Work out the finished part from the listing and answer in its coordinate system (mm). A direction names the side the tool comes from. Round coordinates to 2 decimals unless told otherwise and drop trailing zeros. Write each loop counter-clockwise with the first axis right and the second up, starting at its lowest first coordinate (ties: lowest second). Pieces come first, ordered by that corner, then holes. Notation, with made-up numbers: (-32.5, 19) -> (21.5, 19) arc R19 ccw to (21.5, 35) -> close; hole circle Ø8 at (-27.5, 58.25). An arc over 180 degrees is marked (long way). Answer as a JSON object with one key per item and string values. Group by question number.
from build123d import *

# Parameters (mm, degrees)
F1_DEPTH = 19.05
F3_D     = 12.7
F5_D     = 12.7
F6_R     = 2.54


with BuildPart() as f1:
    # F0 (on Top) → F1 (new body)
    with BuildSketch(Plane.XY):
        Polygon((45.404016, -4.03813), (-1.694917, -4.03813), (-1.694917, 5.48687), (-33.444917, 5.48687), (-33.444917, -0.86313), (-7.148128, -0.86313), (-7.148128, -26.26313), (-33.444917, -26.26313), (-33.444917, -32.61313), (-1.694917, -32.61313), (-1.694917, -23.08813), (45.404016, -23.08813), align=None)
    extrude(amount=F1_DEPTH)

    # F3 (through all)
    with Locations(Plane.XZ.offset(32.61313)):
        with Locations((-23.919917, 9.525)):
            Hole(F3_D / 2)

    # F5 (through all)
    with Locations(Plane.XZ.offset(23.08813)):
        with Locations((35.879016, 9.525)):
            Hole(F5_D / 2)

    # F6
    f6_edges = [f1.edges().sort_by_distance(p)[0] for p in [
        (45.404016, -13.56313, 19.05),
        (45.404016, -13.56313, 0),
        (-7.148128, -13.56313, 19.05),
        (-7.148128, -13.56313, 0),
    ]]
    fillet(f6_edges, radius=F6_R)


solid = f1.part
1) A cutting plane is placed at C-C on y = -18. Determine the outline of the cut face in (x, z) (3 decimals), plus the area to 3 significant figures.
2) Each of these flat-tipped pins is pushed along its axis until it touches: P1, Ø5, axis at x = 25.5, z = 10, coming from the -Y side; P2, Ø7, axis at y = -9, z = 7, coming from the -X side; P3, Ø5.5, axis at x = -25, z = 8.5, coming from the +Y side; P4, Ø3, axis at y = -28, z = 13.5, coming from the +X side. Where does it stop, or does it pass through?
3) A cutting plane is placed at D-D on x = 20. Determine the outline of the cut face in (y, z).
4) A tool of negligible diameter and unlimited length cuts with its end or side. For faces 4 (the face through (-6.38, -13.74, 18.33)), 5 (the face through (22, -4.038, 9)), 6 (the face through (-1.695, -28, 9)), from which of +Z, -Z, +X, -X, +Y, -Y can it reach the whole face along a straight path? Write none if from no direction.
5) Straight lines are drawn through the part: L1, parallel to Y at x = -12, z = 1.5; L2, parallel to Y at x = 0.5, z = 16.5; L3, parallel to X at y = -21, z = 3.75. For each, find the intervals that lie inside material, in ascending order.
6) A cutting plane is placed at A-A on x = -15. Determine the outline of the cut face in (y, z), plus the area to 3 significant figures.
7) A cutting plane is placed at B-B on z = 13.5. Determine the outline of the cut face in (x, y).
8) For a pull along Y with two mould halves and no side action, classify faces 1 (the face through (-14, -32.613, 9)), 2 (the face through (-7.148, -13, 9)), 3 (the face through (44.68, -13.43, 0.764)) as released by +Y, released by -Y, zero draft, split by the parting line, or undercut.
Established:
{
 "1": {"outline": "(-7.148, 2.54) arc R2.54 ccw to (-4.608, 0) -> (42.864, 0) arc R2.54 ccw to (45.404, 2.54) -> (45.404, 16.51) arc R2.54 ccw to (42.864, 19.05) -> (-4.608, 19.05) arc R2.54 ccw to (-7.148, 16.51) -> close; hole circle Ø12.7 at (35.879, 9.525)", "area": "869 mm²"},
 "2": {"P1": "stops at y = -23.09", "P2": "stops at x = -7.15", "P3": "passes through", "P4": "stops at x = -1.69"},
 "3": {"outline": "(-23.09, 0) -> (-4.04, 0) -> (-4.04, 19.05) -> (-23.09, 19.05) -> close"},
 "4": {"face 4": "+Z, -X", "face 5": "+Z, -Z, +X, +Y", "face 6": "+Z, -Z, +X, -Y"},
 "5": {"L1": "y = -32.61 to -26.26, -0.86 to 5.49", "L2": "y = -23.09 to -4.04", "L3": "x = -7.15 to 33.24, 38.52 to 45.4"},
 "6": {"outline": "(-32.61, 0) -> (-26.26, 0) -> (-26.26, 19.05) -> (-32.61, 19.05) -> close; (-0.86, 0) -> (5.49, 0) -> (5.49, 19.05) -> (-0.86, 19.05) -> close", "area": "242 mm²"},
 "7": {"outline": "(-33.44, -32.61) -> (-28.87, -32.61) -> (-28.87, -26.26) -> (-33.44, -26.26) -> close; (-33.44, -0.86) -> (-28.87, -0.86) -> (-28.87, 5.49) -> (-33.44, 5.49) -> close; (-18.97, -32.61) -> (-1.69, -32.61) -> (-1.69, -23.09) -> (30.93, -23.09) -> (30.93, -4.04) -> (-1.69, -4.04) -> (-1.69, 5.49) -> (-18.97, 5.49) -> (-18.97, -0.86) -> (-7.15, -0.86) -> (-7.15, -26.26) -> (-18.97, -26.26) -> close; (40.83, -23.09) -> (45.4, -23.09) -> (45.4, -4.04) -> (40.83, -4.04) -> close"},
 "8": {"face 1": "released by -Y", "face 2": "undercut", "face 3": "zero draft"}
}
